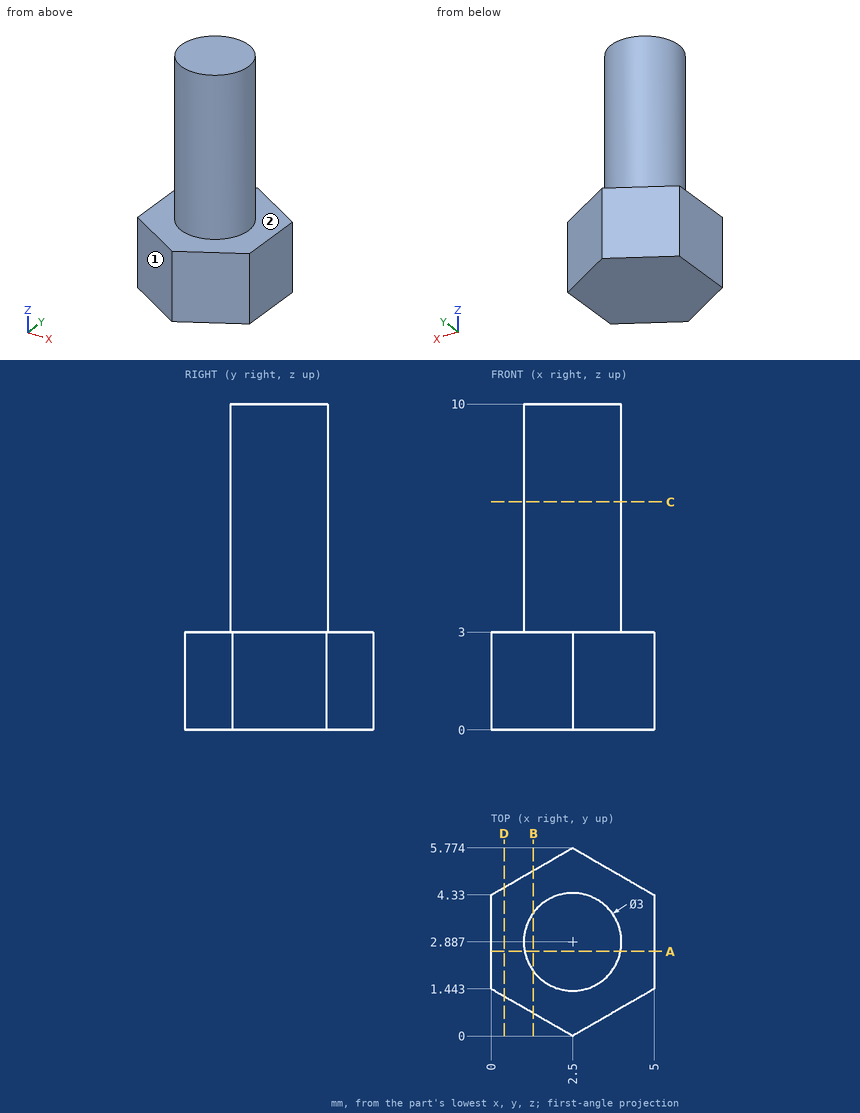
Study the drawing (mm; zero at the part's minimum x, y, z) and answer. A direction names the side the tool comes from. Give positions to 0.01 mm unless a question says otherwise; leave off trailing zeros. Loops run counter-clockwise (first coordinate to the right, second up) from the corner with the lowest first, then second, coordinate; pieces in that order, holes last. Notation, with made-up numbers: (-8, 56) - (15, 56) arc R18 cw to (15, 86) - close; hole circle Ø2 at (15.5, -30.75). An arc over 180 degrees is marked (long way). Return JSON: item names as keys, results as strings. Group by question number.
1. Which of the six approach directions +Z, -Z, +X, -X, +Y, -Y give full straight-line access (tool end or side, diameter ignored) to the marked faces 1 and 2?
2. Find section C-C (z = 7). Write down the section's boundary in (x, y).
3. Given pin 1 Ø1.5 at (y, z) = (3, 2) entering from -X, flat-ended and moving along its own axis, determine where the tip first touches the part or whether it passes through.
4. Find section B-B (x = 1.3). Write down the section's boundary in (y, z).
5. Find section D-D (x = 0.4). Write down the section's boundary in (y, z).
6. Find section A-A (y = 2.6). Write down the section's boundary in (x, z), then the cut area to 3 significant figures.
7. Straight lines are drawn through the part: line 1 (Z direction, x = 1.25, y = 2); line 2 (Y direction, x = 2.1, z = 5); line 3 (Y direction, x = 1.2, z = 7.25) (1 decimal). For each, find the intervals that lie inside material, in ascending order. Write a range as [from, to].
Verdict:
{
 "1": {"face 1": "+Z, -Z, -X, -Y", "face 2": "+Z"},
 "2": {"outline": "circle Ø3 at (2.5, 2.89)"},
 "3": {"pin 1": "stops at x = 0"},
 "4": {"outline": "(0.69, 0) - (5.08, 0) - (5.08, 3) - (3.79, 3) - (3.79, 10) - (1.99, 10) - (1.99, 3) - (0.69, 3) - close"},
 "5": {"outline": "(1.21, 0) - (4.56, 0) - (4.56, 3) - (1.21, 3) - close"},
 "6": {"outline": "(0, 0) - (5, 0) - (5, 3) - (3.97, 3) - (3.97, 10) - (1.03, 10) - (1.03, 3) - (0, 3) - close", "area": "35.6 mm^2"},
 "7": {"line 1": "z = [0, 3]", "line 2": "y = [1.44, 4.33]", "line 3": "y = [2.1, 3.6]"}
}
